Source: CAD feature listing. Evaluate the final solid. Frame: model axes, mm. Round coordinates to 2 decimals unless told otherwise and drop trailing zeros. Loops run counter-clockwise (first coordinate to the right, second up) from the corner with the lowest first, then second, coordinate; pieces in that order, holes last. Notation, with made-up numbers: M 40,-39 L 50,-39 A8 ccw 50,-26 Z; hole C -4,73.25 d7. An arc over 180 degrees is marked long. Answer as a JSON object with one key per item and string values.
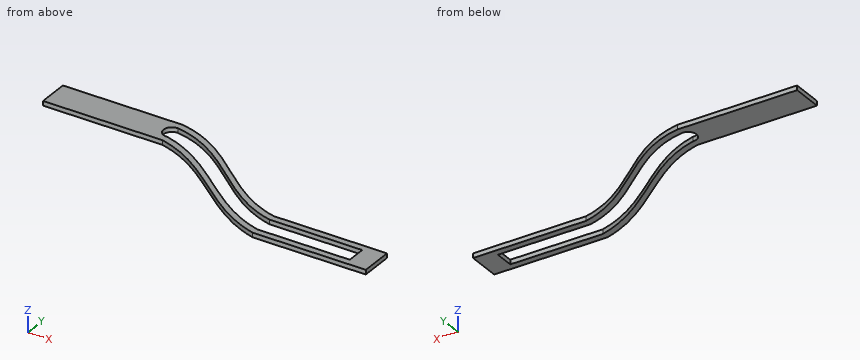
from build123d import *

# Parameters (mm, degrees)
BOSS_EXTRUDE1_DEPTH = 3.8


with BuildPart() as part:
    # Sketch1 → Boss-Extrude1 (new body)
    with BuildSketch(Plane.XY):
        with BuildLine():
            Line((-183.434400527, 71.218162808), (-283.388111119, 71.218162808))
            Line((-283.388111119, 71.218162808), (-283.388111119, 45.671242369))
            Line((-283.388111119, 45.671242369), (-183.434400527, 45.671242369))
            add(Edge.make_bspline(
                [(-183.434400527, 45.671242369), (-135.823073525, 33.710571784), (-108.755954443, -14.312606995), (-60.948326307, -27.25367588)],
                knots=[0, 0, 0, 0, 1, 1, 1, 1], degree=3))
            Line((-60.948326307, -27.25367588), (33.485476227, -27.25367588))
            Line((33.485476227, -27.25367588), (33.485476227, 0))
            Line((33.485476227, 0), (-60.948326307, 0))
            add(Edge.make_bspline(
                [(-183.434400527, 71.218162808), (-134.596760432, 63.241960011), (-109.105838052, 11.434490967), (-60.948326307, 0)],
                knots=[0, 0, 0, 0, 1, 1, 1, 1], degree=3))
        make_face()
        with BuildLine():
            Line((16.41594826, -5.645404289), (-60.948326307, -5.645404289))
            add(Edge.make_bspline(
                [(-183.434400527, 65.418162808), (-134.494216102, 57.813087075), (-109.135947228, 5.64820533), (-60.948326307, -5.645404289)],
                knots=[0, 0, 0, 0, 1, 1, 1, 1], degree=3))
            ThreePointArc((-183.434400527, 65.418162808), (-191.043377182, 58.444702588), (-183.434400527, 51.471242369))
            add(Edge.make_bspline(
                [(-183.434400527, 51.471242369), (-135.942087972, 39.160056631), (-108.723006617, -8.535375407), (-60.948326307, -21.608271591)],
                knots=[0, 0, 0, 0, 1, 1, 1, 1], degree=3))
            Line((-60.948326307, -21.608271591), (16.41594826, -21.608271591))
            Line((16.41594826, -21.608271591), (16.41594826, -5.645404289))
        make_face(mode=Mode.SUBTRACT)
    extrude(amount=BOSS_EXTRUDE1_DEPTH)


solid = part.part
Item 1: Section A-A on x = -52. Return the cut outline in (y, z).
Answer sheet:
{"outline": "M -27.25,0 L -21.61,0 L -21.61,3.8 L -27.25,3.8 Z; M -5.65,0 L 0,0 L 0,3.8 L -5.65,3.8 Z"}
Item 2: Line query: probe 1 along Y at (x, z) = (-48.5, 2.3); probe 2 along Y at (x, z) = (-244, 0.4); probe 3 along Y at (x, z) = (-86.5, 2.4). Output: solid intervals per line, ascending. Write a range as from..to.
Answer sheet:
{"probe 1": "y = -27.25..-21.61, -5.65..0", "probe 2": "y = 45.67..71.22", "probe 3": "y = -16.41..-10.73, 4.77..10.45"}
Item 3: Contact query for flat-ended pins moving along their axis: pin 1 Ø1.5 at (y, z) = (30, 1) entering from +X; pin 2 Ø1.9 at (x, z) = (1, 1.5) entering from +Y; pin 3 Ø1.9 at (x, z) = (-239.5, 1.5) entering from -Y. Output: stop coordinate, or through.
Answer sheet:
{"pin 1": "stops at x = -112.69", "pin 2": "stops at y = 0", "pin 3": "stops at y = 45.67"}
Item 4: Section B-B on x = -212.5. Return the cut outline in (y, z), then the cut area to 3 significant figures.
Answer sheet:
{"outline": "M 45.67,0 L 71.22,0 L 71.22,3.8 L 45.67,3.8 Z", "area": "97.1 mm²"}
